For this review, take the finished solid that the model builds, in its own axes (mm). Face numbers are marked on the shaded views. A direction names the side the tool comes from. Coordinates: 2 decimals unless noted, no trailing zeros. Write each loop counter-clockwise with the first axis right and the second up, starting at its lowest first coordinate (ties: lowest second). Pieces come first, ordered by that corner, then holes. Notation, with made-up numbers: M 24.25,34 L 79.25,34 A28 cw 79.25,54 Z; hole C 79.25,57.5 d9. An arc over 180 degrees is marked long. One line per question, with ' | ' between items.
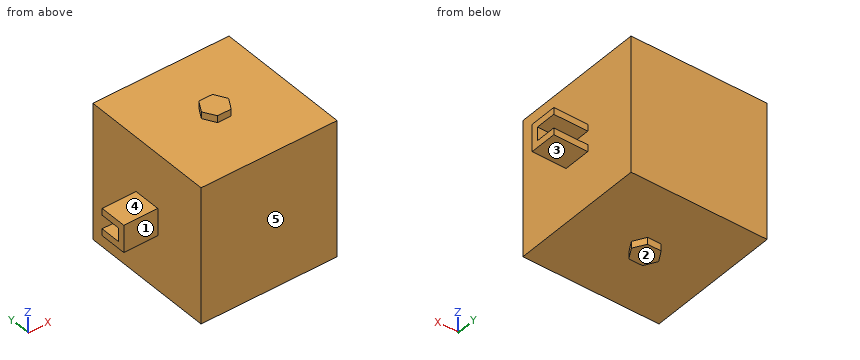
from build123d import *

# Parameters (mm, degrees)
SKETCH1_W           = 50
SKETCH1_H           = 50
BOSS_EXTRUDE1_DEPTH = 50
SKETCH2_W           = 5
SKETCH2_H           = 5
BOSS_EXTRUDE2_DEPTH = 12.5
SKETCH3_W           = 5
SKETCH3_H           = 7.5
CUT_EXTRUDE1_DEPTH  = 12.5
SKETCH6_W           = 10
SKETCH6_H           = 10
BOSS_EXTRUDE3_DEPTH = 12.5
SKETCH7_W           = 5
SKETCH7_H           = 7.5
CUT_EXTRUDE2_DEPTH  = 12.5
BOSS_EXTRUDE5_DEPTH = 2.5
BOSS_EXTRUDE6_DEPTH = 2.5


with BuildPart() as part:
    # Sketch1 → Boss-Extrude1 (new body)
    with BuildSketch(Plane.XY):
        Rectangle(SKETCH1_W, SKETCH1_H)
    extrude(amount=BOSS_EXTRUDE1_DEPTH)

    # Sketch2 → Boss-Extrude2 (add)
    with BuildSketch(Plane.ZY.offset(25)):
        with Locations((27.5, -2.5)):
            Rectangle(SKETCH2_W, SKETCH2_H)
        with Locations((22.5, -2.5)):
            Rectangle(SKETCH2_W, SKETCH2_H)
        with Locations((22.5, 2.5)):
            Rectangle(SKETCH2_W, SKETCH2_H)
        with Locations((27.5, 2.5)):
            Rectangle(SKETCH2_W, SKETCH2_H)
    extrude(amount=BOSS_EXTRUDE2_DEPTH)

    # Sketch3 → Cut-Extrude1 (cut)
    with BuildSketch(Plane.ZY.offset(37.5)):
        with Locations((25, 1.25)):
            Rectangle(SKETCH3_W, SKETCH3_H)
    extrude(amount=-CUT_EXTRUDE1_DEPTH, mode=Mode.SUBTRACT)

    # Sketch6 → Boss-Extrude3 (add)
    with BuildSketch(Plane(origin=(25, 0, 0), x_dir=(0, 0, -1), z_dir=(1, 0, 0))):
        with Locations((-25, 0)):
            Rectangle(SKETCH6_W, SKETCH6_H)
    extrude(amount=BOSS_EXTRUDE3_DEPTH)

    # Sketch7 → Cut-Extrude2 (cut)
    with BuildSketch(Plane(origin=(37.5, 0, 0), x_dir=(0, 0, -1), z_dir=(1, 0, 0))):
        with Locations((-25, 1.25)):
            Rectangle(SKETCH7_W, SKETCH7_H)
    extrude(amount=-CUT_EXTRUDE2_DEPTH, mode=Mode.SUBTRACT)

    # Sketch16 → Boss-Extrude5 (add)
    with BuildSketch(Plane.XY.offset(50)):
        Polygon((5, 0), (2.5, 4.330127019), (-2.5, 4.330127019), (-5, 0), (-2.5, -4.330127019), (2.5, -4.330127019), align=None)
    extrude(amount=BOSS_EXTRUDE5_DEPTH)

    # Sketch17 → Boss-Extrude6 (add)
    with BuildSketch(Plane(origin=(0, 0, 0), x_dir=(-1, 0, 0), z_dir=(0, 0, -1))):
        Polygon((5, 0), (2.5, 4.330127019), (-2.5, 4.330127019), (-5, 0), (-2.5, -4.330127019), (2.5, -4.330127019), align=None)
    extrude(amount=BOSS_EXTRUDE6_DEPTH)


solid = part.part
1) Machinability: for the marked faces 1, 2, 3, 4 and 5, which of the approach directions +Z, -Z, +X, -X, +Y, -Y give a long, thin tool a straight path to every point of the face, cutting with its end or side? Answer none if there is none.
Responses:
face 1: +Z, -Z, -X, -Y | face 2: -Z, +X, -X, +Y, -Y | face 3: -Z, +X, +Y, -Y | face 4: +Z, -X, +Y, -Y | face 5: +Z, -Z, +X, -X, -Y
2) We need section C-C on y = 8. State the section outline as (x, z) points, then the cut area to 3 significant figures.
Responses:
outline: M -25,0 L 25,0 L 25,50 L -25,50 Z | area: 2,500 mm^2
3) To check wall thickness, follow line 1 along Z through (x, y) = (28, 1); line 2 along X through (y, z) = (4, 37); line 3 along Z through (x, y) = (-2, -17). State the ranges of each line that lie inside material, in increasing order. Write a range as [from, to].
Responses:
line 1: [20, 22.5], [27.5, 30] | line 2: [-25, 25] | line 3: [0, 50]
4) We need section B-B on z = 21.5. State the section outline as (x, y) points.
Responses:
outline: M -37.5,-5 L -25,-5 L -25,-25 L 25,-25 L 25,-5 L 37.5,-5 L 37.5,5 L 25,5 L 25,25 L -25,25 L -25,5 L -37.5,5 Z
5) We need section D-D on z = 34.5. State the section outline as (x, y) points.
Responses:
outline: M -25,-25 L 25,-25 L 25,25 L -25,25 Z
6) We need section A-A on x = 31.5. State the section outline as (y, z) points, then the cut area to 3 significant figures.
Responses:
outline: M -5,20 L 5,20 L 5,22.5 L -2.5,22.5 L -2.5,27.5 L 5,27.5 L 5,30 L -5,30 Z | area: 62.5 mm^2
7) Insertion check: pin 1 Ø1.5 at (y, z) = (17, 44.5) entering from -X; pin 2 Ø4 at (x, z) = (30.5, 25) entering from +Y; pin 3 Ø6 at (x, y) = (-33.5, 3) entering from +Z. Each pin has a flat end and moves straight along its axis. Give the tip position at first contact, or say it passes through.
Responses:
pin 1: x = -25 | pin 2: y = -2.5 | pin 3: z = 30
